Source: three-view drawing plus pictorial views. Frame: mm from the lowest corner of the part. A direction names the side the tool comes from. Give positions to 0.01 mm unless a question says otherwise; leave off trailing zeros. Loops run counter-clockwise (first coordinate to the right, second up) from the corner with the lowest first, then second, coordinate; pieces in that order, holes last.
1. Section A-A, the plane x = 11.25. Output: boundary loops of the cut face in (y, z).
2. First-contact query: P1, Ø11, axis at x = 91, y = 13, coming from the -Z side; P2, Ø7, axis at x = 84.5, y = 3, coming from the +Z side; P3, Ø2, axis at x = 85, y = 4, coming from the -Z side; P4, Ø3, axis at y = 4, z = 25, coming from the -X side. Flat tips, straight axial feed; report the tip coordinate or a pass-through.
3. Draft query along X for the marked faces 1, 2, 3 and 4. Return one class per face: +X half, -X half, draft (parallel to the pull), parting line (faces both ways), or undercut.
4. Access query for the marked faces 5, 6 and 7. Directions: +Z, -Z, +X, -X, +Y, -Y. A direction counts if a zero-diameter tool reaches every point of the face in a straight line with its end or side. Return the directions, or none.
5. Material intervals for line 1 along Y through (x, z) = (11.25, 32.75); line 2 along Y through (x, z) = (63.5, 8); line 3 along Y through (x, z) = (93, 31) (1 decimal), sorted ascending.
6. Section D-D, the plane z = 21. Output: boundary loops of the cut face in (x, y) (1 decimal), then the cut area to 3 significant figures.
7. Section C-C, the plane z = 31. Output: boundary loops of the cut face in (x, y).
8. Section B-B, the plane y = 4. Output: boundary loops of the cut face in (x, z) (1 decimal).
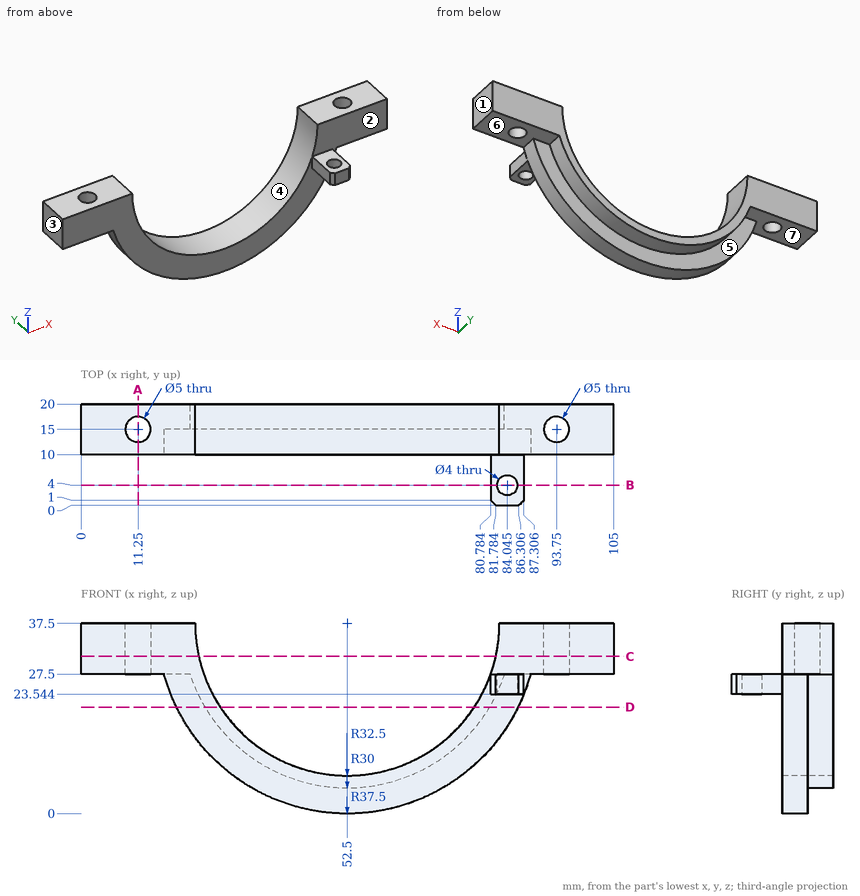
Answers below:
1. outline: (10, 27.5) - (12.5, 27.5) - (12.5, 37.5) - (10, 37.5) - close; (17.5, 27.5) - (20, 27.5) - (20, 37.5) - (17.5, 37.5) - close
2. P1: stops at z = 19.69
2. P2: stops at z = 27.5
2. P3: passes through
2. P4: stops at x = 80.78
3. face 1: +X half
3. face 2: draft
3. face 3: -X half
3. face 4: undercut
4. face 5: -Z, +Y
4. face 6: -Z, +X, +Y
4. face 7: -Z, -X, +Y
5. line 1: y = 10 to 12.5, 17.5 to 20
5. line 2: y = 10 to 20
5. line 3: y = 10 to 12.6, 17.4 to 20
6. outline: (18.8, 10) - (27.4, 10) - (27.4, 20) - (24.5, 20) - (24.5, 15) - (18.8, 15) - close; (77.6, 10) - (86.2, 10) - (86.2, 15) - (80.5, 15) - (80.5, 20) - (77.6, 20) - close
6. area: 116 mm2
7. outline: (0, 10) - (23.21, 10) - (23.21, 20) - (0, 20) - close; (81.79, 10) - (105, 10) - (105, 20) - (81.79, 20) - close; hole circle Ø5 at (11.25, 15); hole circle Ø5 at (93.75, 15)
8. outline: (80.8, 23.5) - (82, 23.5) - (82, 27.5) - (80.8, 27.5) - close; (86, 23.5) - (87.3, 23.5) - (87.3, 27.5) - (86, 27.5) - close
